from build123d import *

# Parameters (mm, degrees)
SKETCH_2_W           = 65.2997206
SKETCH_2_H           = 38
SKETCH_2_R           = 1.00000254
SKETCH_2_R_2         = 0.922218434
SKETCH_2_R_3         = 1.5
EXTRUDE_2_DEPTH      = 4.5
SKETCH_3_R           = 1.5
CUT_EXTRUDE_2_DEPTH  = 2.5
SKETCH_5_W           = 65.2997206
SKETCH_5_H           = 38
SKETCH_5_W_2         = 61.2997206
SKETCH_5_H_2         = 34
EXTRUDE_3_DEPTH      = 21
EXTRUDE_3_DEPTH_BACK = 16
SKETCH_7_W           = 8.214112973
SKETCH_7_H           = 3.795011114
CUT_EXTRUDE_4_DEPTH  = 3
SKETCH_8_W           = 4
SKETCH_8_H           = 9.575559499
CUT_EXTRUDE_5_DEPTH  = 3
SKETCH_9_W           = 9.326303795
SKETCH_9_H           = 4.202278939
CUT_EXTRUDE_6_DEPTH  = 3
CUT_EXTRUDE_7_DEPTH  = 10
SKETCH_15_R          = 1.75
CUT_EXTRUDE_8_DEPTH  = 1.5
SKETCH_18_W          = 62.2997206
SKETCH_18_H          = 36
CUT_EXTRUDE_9_DEPTH  = 3
SKETCH_19_W          = 3
SKETCH_19_H          = 6
CUT_EXTRUDE_10_DEPTH = 2
SKETCH_20_W          = 2
SKETCH_20_H          = 8
CUT_EXTRUDE_11_DEPTH = 3
SKETCH_21_W          = 4.5
SKETCH_21_H          = 8
EXTRUDE_4_DEPTH      = 8
SKETCH_22_R          = 1.5
CUT_EXTRUDE_12_DEPTH = 10
CUT_EXTRUDE_13_DEPTH = 2.5
FILLET_1_R           = 1


with BuildPart() as part:
    # 草图2 → 凸台-拉伸2 (new body)
    with BuildSketch(Plane(origin=(0, 0, -6), x_dir=(-1, 0, 0), z_dir=(0, 0, -1))):
        with Locations((29.273558547, -24.066548133)):
            Rectangle(SKETCH_2_W, SKETCH_2_H)
        with Locations((1.016002032, -11.24978156)):
            Circle(SKETCH_2_R, mode=Mode.SUBTRACT)
        with Locations((0.889001778, -36.83007366)):
            Circle(SKETCH_2_R, mode=Mode.SUBTRACT)
        with Locations((57.658115316, -36.64983236)):
            Circle(SKETCH_2_R, mode=Mode.SUBTRACT)
        with Locations((57.658115316, -11.24978156)):
            Circle(SKETCH_2_R_2, mode=Mode.SUBTRACT)
        with Locations((29.273558547, -32.316548133)):
            Circle(SKETCH_2_R_3, mode=Mode.SUBTRACT)
        with BuildLine():
            Line((27.785407033, -15.816548133), (27.785407033, -13.183619987))
            ThreePointArc((27.785407033, -13.183619987), (29.273558547, -11.695468472), (30.761710061, -13.183619987))
            Line((30.761710061, -13.183619987), (30.761710061, -15.816548133))
            ThreePointArc((30.761710061, -15.816548133), (29.273558547, -17.304699647), (27.785407033, -15.816548133))
        make_face(mode=Mode.SUBTRACT)
    extrude(amount=EXTRUDE_2_DEPTH)

    # 草图3 → 切除-拉伸2 (cut)
    with BuildSketch(Plane(origin=(0, 0, -6), x_dir=(-1, 0, 0), z_dir=(0, 0, -1))):
        Polygon((29.273558547, -18.991974614), (32.023558547, -17.404261373), (32.023558547, -14.920341582), (32.023558547, -14.228834893), (32.023558547, -11.744915102), (29.273558547, -10.157201862), (26.523558547, -11.744915102), (26.523558547, -14.228834893), (26.523558547, -14.920341582), (26.523558547, -17.404261373), align=None)
        with BuildLine():
            ThreePointArc((30.761710061, -15.816548133), (29.273558547, -17.304699647), (27.785407033, -15.816548133))
            Line((27.785407033, -15.816548133), (27.785407033, -13.183619987))
            ThreePointArc((27.785407033, -13.183619987), (29.273558547, -11.695468472), (30.761710061, -13.183619987))
            Line((30.761710061, -13.183619987), (30.761710061, -15.816548133))
        make_face(mode=Mode.SUBTRACT)
        Polygon((26.523558547, -30.728834893), (26.523558547, -33.904261373), (29.273558547, -35.491974614), (32.023558547, -33.904261373), (32.023558547, -30.728834893), (29.273558547, -29.141121653), align=None)
        with Locations((29.273558547, -32.316548133)):
            Circle(SKETCH_3_R, mode=Mode.SUBTRACT)
    extrude(amount=CUT_EXTRUDE_2_DEPTH, mode=Mode.SUBTRACT)

    # 草图5 → 凸台-拉伸3 (add, two sides)
    with BuildSketch(Plane(origin=(0, 0, -10.5), x_dir=(-1, 0, 0), z_dir=(0, 0, -1))) as extrude_3_sk:
        with Locations((29.273558547, -24.066548133)):
            Rectangle(SKETCH_5_W, SKETCH_5_H)
        with Locations((29.273558547, -24.066548133)):
            Rectangle(SKETCH_5_W_2, SKETCH_5_H_2, mode=Mode.SUBTRACT)
    extrude(amount=EXTRUDE_3_DEPTH)
    extrude(extrude_3_sk.sketch, amount=-EXTRUDE_3_DEPTH_BACK)

    # 草图7 → 切除-拉伸4 (cut)
    with BuildSketch(Plane(origin=(0, -5.066548133, 0), x_dir=(1, 0, 0), z_dir=(0, 1, 0))):
        with Locations((-50.955145133, -3.662545243)):
            Rectangle(SKETCH_7_W, SKETCH_7_H)
    extrude(amount=-CUT_EXTRUDE_4_DEPTH, mode=Mode.SUBTRACT)

    # 草图8 → 切除-拉伸5 (cut)
    with BuildSketch(Plane.ZY.offset(61.923418847)):
        with Locations((3.6000508, -23.483057223)):
            Rectangle(SKETCH_8_W, SKETCH_8_H)
    extrude(amount=-CUT_EXTRUDE_5_DEPTH, mode=Mode.SUBTRACT)

    # 草图9 → 切除-拉伸6 (cut)
    with BuildSketch(Plane.XZ.offset(43.066548133)):
        with Locations((-44.464129124, 3.49891133)):
            Rectangle(SKETCH_9_W, SKETCH_9_H)
    extrude(amount=-CUT_EXTRUDE_6_DEPTH, mode=Mode.SUBTRACT)

    # 草图13 → 切除-拉伸7 (cut)
    with BuildSketch(Plane.XY.offset(-6)):
        Polygon((-59.923418847, -16.066514367), (-59.923418847, -19.252115931), (-54.525349934, -19.252115931), (-54.525349934, -41.066548133), (-34.525349934, -41.066548133), (-34.525349934, -7.066548133), (-54.525349934, -7.066548133), (-54.525349934, -12.880912803), (-54.525349934, -16.066514367), align=None)
    extrude(amount=-CUT_EXTRUDE_7_DEPTH, mode=Mode.SUBTRACT)

    # 草图15 → 切除-拉伸8 (cut)
    with BuildSketch(Plane(origin=(0, 0, -10.5), x_dir=(-1, 0, 0), z_dir=(0, 0, -1))):
        with Locations((1.016002032, -11.24978156)):
            Circle(SKETCH_15_R)
        with Locations((57.658115316, -11.24978156)):
            Circle(SKETCH_15_R)
        with Locations((0.889001778, -36.83007366)):
            Circle(SKETCH_15_R)
        with Locations((57.658115316, -36.64983236)):
            Circle(SKETCH_15_R)
    extrude(amount=-CUT_EXTRUDE_8_DEPTH, mode=Mode.SUBTRACT)

    # 草图18 → 切除-拉伸9 (cut)
    with BuildSketch(Plane(origin=(0, 0, -31.5), x_dir=(-1, 0, 0), z_dir=(0, 0, -1))):
        with Locations((29.773558547, -24.066548133)):
            Rectangle(SKETCH_18_W, SKETCH_18_H)
    extrude(amount=-CUT_EXTRUDE_9_DEPTH, mode=Mode.SUBTRACT)

    # 草图19 → 切除-拉伸10 (cut)
    with BuildSketch(Plane.ZY.offset(-1.376301753)):
        with Locations((-28, -10.066548133)):
            Rectangle(SKETCH_19_W, SKETCH_19_H)
        with Locations((-28, -38.066548133)):
            Rectangle(SKETCH_19_W, SKETCH_19_H)
    extrude(amount=-CUT_EXTRUDE_10_DEPTH, mode=Mode.SUBTRACT)

    # 草图20 → 切除-拉伸11 (cut)
    with BuildSketch(Plane(origin=(0, 0, -31.5), x_dir=(-1, 0, 0), z_dir=(0, 0, -1))):
        with Locations((60.923418847, -24.066548133)):
            Rectangle(SKETCH_20_W, SKETCH_20_H)
    extrude(amount=-CUT_EXTRUDE_11_DEPTH, mode=Mode.SUBTRACT)

    # 草图21 → 凸台-拉伸4 (add)
    with BuildSketch(Plane.ZY.offset(61.923418847)):
        with Locations((-26.25, -24.066548133)):
            Rectangle(SKETCH_21_W, SKETCH_21_H)
    extrude(amount=EXTRUDE_4_DEPTH)

    # 草图22 → 切除-拉伸12 (cut)
    with BuildSketch(Plane.XY.offset(-24)):
        with Locations((-65.923418847, -24.066548133)):
            Circle(SKETCH_22_R)
    extrude(amount=-CUT_EXTRUDE_12_DEPTH, mode=Mode.SUBTRACT)

    # 草图23 → 切除-拉伸13 (cut)
    with BuildSketch(Plane.XY.offset(-24)):
        Polygon((-64.335705607, -26.816548133), (-62.747992366, -24.066548133), (-64.335705607, -21.316548133), (-67.511132087, -21.316548133), (-69.098845327, -24.066548133), (-67.511132087, -26.816548133), align=None)
    extrude(amount=-CUT_EXTRUDE_13_DEPTH, mode=Mode.SUBTRACT)

    # 圆角1
    fillet_1_edges = [part.edges().sort_by_distance(p)[0] for p in [
        (-69.923418847, -28.066548133, -26.25),
        (-69.923418847, -20.066548133, -26.25),
    ]]
    fillet(fillet_1_edges, radius=FILLET_1_R)


solid = part.part
The listing builds one solid part. Answer for the finished solid, in the listing's coordinates (mm). A direction names the side the tool comes from. Round coordinates to 2 decimals unless told otherwise and drop trailing zeros. Write each loop counter-clockwise with the first axis right and the second up, starting at its lowest first coordinate (ties: lowest second). Pieces come first, ordered by that corner, then holes. Notation, with made-up numbers: M 43,7 L 88,7 A8 ccw 88,14 Z; hole C -15,40.25 d4. An arc over 180 degrees is marked long. Write each question's results on one line, items separated by ' | '. Start each with the question number.
Item 1: Straight lines are drawn through the part: probe 1 along X at (y, z) = (-28, -3.5); probe 2 along Y at (x, z) = (-17.5, -13); probe 3 along X at (y, z) = (-14, -29). For each, find the intervals that lie inside material, in ascending order.
Item 2: Find section D-D on x = -7. Write down the section's boundary in (y, z).
Item 3: Which of the six approach directions +Z, -Z, +X, -X, +Y, -Y give full straight-line access (tool end or side, diameter ignored) to faces 1 (the flat face through (-65, -28.067, -26)), 2 (the flat face through (-32.024, -15, -7)), 3 (the flat face through (-55.062, -6, 4)), 4 (the flat face through (2, -35.067, -28)), 5 (the flat face through (-60.923, -13, -30))?
Item 4: The mould has two halves that part along X. Classify faces 6 (the flat face through (-30.668, -10.962, -7.232)), 7 (the flat face through (2, -10, -26.5)): +X half, -X half, draft (parallel to the pull), parting line (faces both ways), or undercut.
Item 5: Find section B-B on x = -52.5. Write down the section's boundary in (y, z), and give its area (3 significant figures).
Item 6: Given pin 1 Ø1.6 at (x, y) = (-61.5, -24.5) entering from +Z; pin 2 Ø1.3 at (y, z) = (-19, -8) entering from -X; pin 3 Ø6 at (x, y) = (-23.5, -25.5) entering from +Z, each flat-ended and moving along its own axis, determine where each tip first touches the part or whether it passes through.
Item 7: Find section A-A on y = -14. Write down the section's boundary in (x, z), and give its area (3 significant figures).
Item 8: Find section C-C on z = -14. Write down the section's boundary in (x, y), and give its area (3 significant figures).
Answer block:
1) probe 1: x = -61.92 to -59.92, 1.38 to 3.38 | probe 2: y = -43.07 to -41.07, -7.07 to -5.07 | probe 3: x = -61.92 to -60.92, 1.38 to 3.38
2) outline: M -43.07,-31.5 L -42.07,-31.5 L -42.07,-28.5 L -41.07,-28.5 L -41.07,-10.5 L -7.07,-10.5 L -7.07,-28.5 L -6.07,-28.5 L -6.07,-31.5 L -5.07,-31.5 L -5.07,5.5 L -7.07,5.5 L -7.07,-6 L -41.07,-6 L -41.07,5.5 L -43.07,5.5 Z
3) face 1: +Z, -Z, -X, -Y | face 2: +Z | face 3: +Z, +Y | face 4: +X | face 5: -Z
4) face 6: undercut | face 7: draft
5) outline: M -43.07,-31.5 L -42.07,-31.5 L -42.07,-28.5 L -41.07,-28.5 L -41.07,5.5 L -43.07,5.5 Z; M -7.07,-28.5 L -6.07,-28.5 L -6.07,-31.5 L -5.07,-31.5 L -5.07,1.77 L -7.07,1.77 Z | area: 135 mm²
6) pin 1: stops at z = 1.6 | pin 2: stops at x = -61.92 | pin 3: stops at z = -6
7) outline: M -61.92,-31.5 L -60.92,-31.5 L -60.92,-28.5 L -59.92,-28.5 L -59.92,-10.5 L -54.53,-10.5 L -54.53,-6 L -59.92,-6 L -59.92,5.5 L -61.92,5.5 Z; M -34.53,-10.5 L -30.76,-10.5 L -30.76,-8.5 L -32.02,-8.5 L -32.02,-6 L -34.53,-6 Z; M -27.79,-10.5 L 1.38,-10.5 L 1.38,-31.5 L 3.38,-31.5 L 3.38,5.5 L 1.38,5.5 L 1.38,-6 L -26.52,-6 L -26.52,-8.5 L -27.79,-8.5 Z | area: 311 mm²
8) outline: M -61.92,-43.07 L 3.38,-43.07 L 3.38,-5.07 L -61.92,-5.07 Z; hole M -59.92,-41.07 L 1.38,-41.07 L 1.38,-7.07 L -59.92,-7.07 Z | area: 397 mm²
